Could you check a few things on this model? Use its own coordinates, in mm. Coordinates: 2 decimals unless noted, no trailing zeros. Loops run counter-clockwise (first coordinate to the right, second up) from the corner with the lowest first, then second, coordinate; pieces in that order, holes last.
1) Imagine slicing it at B-B on y = 23. Please give me the cut outline in (x, z).
2) Will these pins go through, and if not, where does the flat tip stop? P1, Ø1.5, axis at x = -116.5, z = 136, coming from the -Y side; P2, Ø1.2, axis at y = 1, z = 136, coming from the -X side; P3, Ø0.9, axis at x = -117.5, z = 136, coming from the +Y side.
3) If I drill on line 1 along Y through (x, z) = (34, 136.9); line 2 along Y through (x, z) = (-5, 135.7); line 3 along X through (y, z) = (65.5, 135.35), over which ranges is the centre line in solid material (lowest first)?
4) Imagine slicing it at A-A on x = 2.5. Please give me the cut outline in (y, z), plus the area to 3 significant figures.
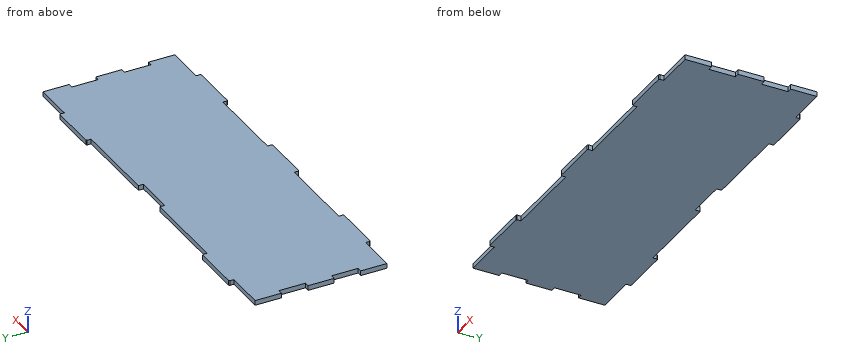
```python
from build123d import *

# Parameters (mm, degrees)
BOSS_EXTRUDE1_DEPTH = 2.9


with BuildPart() as part:
    # Sketch1 → Boss-Extrude1 (new body)
    with BuildSketch(Plane.XY.offset(135)):
        Polygon((-118.9, 2.9), (-95, 2.9), (-95, 0.5), (-94.5, 0), (-65.5, 0), (-65, 0.5), (-65, 2.9), (-15, 2.9), (-15, 0.5), (-14.5, 0), (14.5, 0), (15, 0.5), (15, 2.9), (65, 2.9), (65, 0.5), (65.5, 0), (94.5, 0), (95, 0.5), (95, 2.9), (118.9, 2.9), (118.9, 18.675), (116, 18.675), (116, 34.525), (118.9, 34.525), (118.9, 50.275), (116, 50.275), (116, 66.125), (118.9, 66.125), (118.9, 81.9), (95, 81.9), (95, 84.3), (94.5, 84.8), (65.5, 84.8), (65, 84.3), (65, 81.9), (12, 81.9), (12, 78.9), (-12, 78.9), (-12, 81.9), (-65, 81.9), (-65, 84.3), (-65.5, 84.8), (-94.5, 84.8), (-95, 84.3), (-95, 81.9), (-118.9, 81.9), (-118.9, 66.125), (-116, 66.125), (-116, 50.275), (-118.9, 50.275), (-118.9, 34.525), (-116, 34.525), (-116, 18.675), (-118.9, 18.675), align=None)
    extrude(amount=BOSS_EXTRUDE1_DEPTH)


solid = part.part
```
Filled in:
1. outline: (-116, 135) - (116, 135) - (116, 137.9) - (-116, 137.9) - close
2. P1: stops at y = 2.9
2. P2: stops at x = -95
2. P3: stops at y = 81.9
3. line 1: y = 2.9 to 81.9
3. line 2: y = 0 to 78.9
3. line 3: x = -116 to 116
4. outline: (0, 135) - (78.9, 135) - (78.9, 137.9) - (0, 137.9) - close
4. area: 229 mm2
